Design review of the part built by this model. Coordinates are the model's own, in mm. A direction names the side the tool comes from. Coordinates: 2 decimals unless noted, no trailing zeros. Loops run counter-clockwise (first coordinate to the right, second up) from the corner with the lowest first, then second, coordinate; pieces in that order, holes last. Notation, with made-up numbers: M -3,23.25 L 34,23.25 A20 cw 34,47.25 Z; hole C -29,79.5 d1. An arc over 180 degrees is marked long. One line per item, written item: value.
Autodesk Fusion 360 part; units mm, degrees
sketch "Esquisse1" plane through (0, 0, 0) normal (0, 0, 1) x (1, 0, 0)
  line L0 (71.2, 51.2) -> (-71.2, 51.2)
  line L1 (-71.2, 51.2) -> (-71.2, -21.2)
  line L2 (-71.2, -21.2) -> (71.2, -21.2)
  line L3 (71.2, -21.2) -> (71.2, 51.2)
extrude "Extrusion1" add sketch "Esquisse1" along normal blind 5
extrude "Extrusion2" add 1 faces at (-23.7333, 27.0667, 5) along direction (0, 0, 1) blind 1
sketch "Esquisse2" plane through (0, 0, 6) normal (0, 0, 1) x (-1, 0, 0)
  line L0 (-71.2, 21.2) -> (-71.2, -51.2)
  line L1 (-71.2, -51.2) -> (71.2, -51.2)
  line L2 (71.2, -51.2) -> (71.2, 21.2)
  line L3 (71.2, 21.2) -> (-71.2, 21.2)
  line L4 (70.2, -50.2) -> (-70.2, -50.2)
  line L5 (-70.2, -50.2) -> (-70.2, 20.2)
  line L6 (-70.2, 20.2) -> (70.2, 20.2)
  line L7 (70.2, 20.2) -> (70.2, -50.2)
extrude "Extrusion3" cut sketch "Esquisse2" against normal blind 5 contours L4 L5 L6 L7
sketch "Esquisse3" plane through (0, 0, 1) normal (0, 0, 1) x (-1, 0, 0)
  line L0 (70.2, 20.2) -> (-70.2, 20.2)
  line L1 (-70.2, 20.2) -> (-70.2, -50.2)
  line L2 (-70.2, -50.2) -> (70.2, -50.2)
  line L3 (70.2, -50.2) -> (70.2, 20.2)
  line L4 (45, 0) -> (60, 0)
  line L5 (60, 0) -> (60, -30)
  line L6 (60, -30) -> (45, -30)
  line L7 (45, -30) -> (45, 0)
  line L8 (-60, 0) -> (-45, 0)
  line L9 (-45, 0) -> (-45, -30)
  line L10 (-45, -30) -> (-60, -30)
  line L11 (-60, -30) -> (-60, 0)
extrude "Extrusion4" cut sketch "Esquisse3" against normal blind 1 contours L4 L5 L6 L7 | L8 L9 L10 L11
(1) Tool access review of faces 1 (the flat face through (-1, -21.2, 3)), 2 (the flat face through (-1, 50.2, 4)): name each direction out of +Z, -Z, +X, -X, +Y, -Y from which nothing blocks a thin tool from reaching the whole face with its end or side.
Reply:
face 1: +Z, -Z, +X, -X, -Y
face 2: +Z
(2) Mouldability with a two-part tool opening along X and no side actions: class faces 3 (the flat face through (-71.2, 16, 3)), 4 (the flat face through (71.2, 14, 3)), 5 (the flat face through (1, 15, 1)) as released by +X, released by -X, zero draft, split by the parting line, or undercut.
Reply:
face 3: released by -X
face 4: released by +X
face 5: undercut
(3) To check wall thickness, follow line 1 along Y through (x, z) = (-1, 1.65); line 2 along Y through (x, z) = (52, 0.2); line 3 along X through (y, z) = (40.5, 4). State the ranges of each line that lie inside material, in increasing order. Write a range as [from, to].
Reply:
line 1: y = [-21.2, -20.2], [50.2, 51.2]
line 2: y = [-21.2, 0], [30, 51.2]
line 3: x = [-71.2, -70.2], [70.2, 71.2]
(4) We need section B-B on x = -57. State the section outline as (y, z) points, then the cut area to 3 significant figures.
Reply:
outline: M -21.2,0 L 0,0 L 0,1 L -20.2,1 L -20.2,6 L -21.2,6 Z; M 30,0 L 51.2,0 L 51.2,6 L 50.2,6 L 50.2,1 L 30,1 Z
area: 52.4 mm2
(5) We need section C-C on z = 2.75. State the section outline as (x, y) points.
Reply:
outline: M -71.2,-21.2 L 71.2,-21.2 L 71.2,51.2 L -71.2,51.2 Z; hole M -70.2,-20.2 L 70.2,-20.2 L 70.2,50.2 L -70.2,50.2 Z
(6) We need section A-A on y = 16.5. State the section outline as (x, z) points.
Reply:
outline: M -71.2,0 L -60,0 L -60,1 L -70.2,1 L -70.2,6 L -71.2,6 Z; M -45,0 L 45,0 L 45,1 L -45,1 Z; M 60,0 L 71.2,0 L 71.2,6 L 70.2,6 L 70.2,1 L 60,1 Z
(7) We need section D-D on x = -11. State the section outline as (y, z) points.
Reply:
outline: M -21.2,0 L 51.2,0 L 51.2,6 L 50.2,6 L 50.2,1 L -20.2,1 L -20.2,6 L -21.2,6 Z
(8) Insertion check: pin 1 (2 mm diameter, centred on x = 0.5, y = 23.5, fed in from -Z). The pin has a flat end and moves straight along its axis. Give the tip position at first contact, or say it passes through.
Reply:
pin 1: stops at z = 0
